Autodesk Fusion 360 part; units mm, degrees
sketch "Sketch1" plane through (0, 0, 0) normal (0, 1, 0) x (1, 0, 0)
  line L0 (0, 0) -> (20, 0)
  line L1 (20, 0) -> (20, -112)
  line L2 (20, -112) -> (-59, -112)
  line L3 (-59, -112) -> (-59, -87)
  line L4 (-59, -87) -> (-2.4388, -87)
  line L5 (0, 0) -> (0, -84.5612)
  line L6 (0, -87) -> (1.0607, -88.0607) construction
  line L7 (0, -87) -> (2, -87) construction
  arc A0 (-1.439, -88.0173) -> (1.0173, -85.561) centre (1.0607, -88.0607) ccw
  arc A1 (0, -84.5612) -> (1.0173, -85.561) centre (1, -84.5612) ccw
  arc A2 (-1.439, -88.0173) -> (-2.4388, -87) centre (-2.4388, -88) ccw
  line L8 (-59, -99.5) -> (-49.5, -99.5) construction
  line L9 (-27.9553, -112) -> (-27.9553, -104.5) construction
  line L10 (-27.9553, -87) -> (-27.9553, -94.5) construction
  line L11 (-14.5, -94.5) -> (-44.5, -94.5)
  line L12 (-44.5, -104.5) -> (-14.5, -104.5)
  arc A3 (-14.5, -104.5) -> (-14.5, -94.5) centre (-14.5, -99.5) ccw
  arc A4 (-44.5, -94.5) -> (-44.5, -104.5) centre (-44.5, -99.5) ccw
  point P0 (0, -85.7968)
  dimension "d1" = 20
  dimension "d2" = 112
  dimension "d3" = 79
  dimension "d5" = 59
  dimension "d8" = 45
  dimension "d9" = 1.5
  dimension "d10" = 5
  dimension "d11" = 25
  dimension "d12" = 85.7968
  dimension "d13" = 1
  dimension "d14" = 9.5
  dimension "d15" = 7.5
  dimension "d16" = 7.5
  dimension "d17" = 10
  dimension "d18" = 30
  dimension "d19" = 10
extrude "Extrude1" add sketch "Sketch1" along normal blind 10
sketch "Sketch3" plane through (0, 0, 0) normal (0, 1, 0) x (1, 0, 0)
  line L0 (0, 0) -> (5, 0) construction
  line L1 (5, 0) -> (15, 0)
  line L2 (15, 0) -> (15, -120)
  line L3 (15, -120) -> (5, -120)
  line L4 (5, -120) -> (5, 0)
  dimension "d26" = 5
  dimension "d27" = 10
  dimension "d28" = 120
extrude "Extrude2" cut sketch "Sketch3" along normal blind 0.5
Could you check a few things on this model? Use its own coordinates, in mm. A direction names the side the tool comes from. Round coordinates to 2 decimals unless told otherwise and drop trailing zeros. Loops run counter-clockwise (first coordinate to the right, second up) from the corner with the lowest first, then second, coordinate; pieces in that order, holes last.
Q1. On a 3-axis mill with a long thin cutter (end or side, diameter ignored), from which of +Z, -Z, +X, -X, +Y, -Y can I reach the whole of each face in a straight line? I mean faces 1 (the flat face through (6, 10, 80)), 2 (the cylindrical face through (-9.5, 4.9, 99.4)), 3 (the flat face through (-31, 5, 87)). Say none if no direction works.
Q2. For P1, Ø3, axis at x = 1.06, z = 88.06, coming from the -Y side; P2, Ø4, axis at y = 9, z = 19, coming from the -X side; P3, Ø3, axis at x = 11.5, z = 54, coming from the -Y side; P4, Ø2, axis at x = -33, y = 7, coming from the -Z side, each with a flat end and sliding along its axis, tell me the tip position at first contact or that it passes through.
Q3. Thinking about a two-plate mould opening in X: for faces 4 (the flat face through (10, 0.5, 55)), 5 (the flat face through (-59, 5, 100)), 6 (the flat face through (10, 5, 0)), which applies, pulls with the +X half, pulls with the -X half, needs draft (parallel to the pull), parting line crosses it, or undercut?
Q4. I want a section at B-B (z = 99.5). Write out the boundary of the cut face in (x, y).
Q5. Please list where these lines run through material, in increasing order: L1, parallel to Z at x = -29.5, y = 2.75; L2, parallel to Z at x = -55, y = 3.75; L3, parallel to X at y = 8.5, z = 49.5.
Q6. I want a section at A-A (x = -22). Write out the boundary of the cut face in (y, z).
Q7. I want a section at D-D (y = 4). Write out the boundary of the cut face in (x, z).
Q8. I want a section at C-C (z = 70.5). Write out the boundary of the cut face in (x, y), and give its area (3 significant figures).
Answer below:
1. face 1: +Z, -Z, +X, -X, +Y
1. face 2: +Y, -Y
1. face 3: -Z, -X, +Y, -Y
2. P1: passes through
2. P2: stops at x = 0
2. P3: stops at y = 0.5
2. P4: stops at z = 87
3. face 4: undercut
3. face 5: pulls with the -X half
3. face 6: needs draft
4. outline: (-59, 0) - (-49.5, 0) - (-49.5, 10) - (-59, 10) - close; (-9.5, 0) - (5, 0) - (5, 0.5) - (15, 0.5) - (15, 0) - (20, 0) - (20, 10) - (-9.5, 10) - close
5. L1: z = 87 to 94.5, 104.5 to 112
5. L2: z = 87 to 112
5. L3: x = 0 to 20
6. outline: (0, 87) - (10, 87) - (10, 94.5) - (0, 94.5) - close; (0, 104.5) - (10, 104.5) - (10, 112) - (0, 112) - close
7. outline: (-59, 87) - (-2.44, 87) arc R1 ccw to (-1.44, 88.02) arc R2.5 cw (long way) to (1.02, 85.56) arc R1 ccw to (0, 84.56) - (0, 0) - (20, 0) - (20, 112) - (-59, 112) - close; hole (-44.5, 94.5) - (-14.5, 94.5) arc R5 ccw to (-14.5, 104.5) - (-44.5, 104.5) arc R5 ccw to start
8. outline: (0, 0) - (5, 0) - (5, 0.5) - (15, 0.5) - (15, 0) - (20, 0) - (20, 10) - (0, 10) - close
8. area: 195 mm2
